from build123d import *

# Parameters (mm, degrees)
BOSS_EXTRUDE1_DEPTH = 6
SKETCH3_R           = 1.75
CUT_EXTRUDE1_DEPTH  = 84.570329663
SKETCH4_R           = 1.6
CUT_EXTRUDE2_DEPTH  = 81.721744282
FILLET1_R           = 3
FILLET2_R           = 1


with BuildPart() as part:
    # Sketch2 → Boss-Extrude1 (new body)
    with BuildSketch(Plane(origin=(0, 0, 0), x_dir=(1, 0, 0), z_dir=(0, 1, 0))):
        Polygon((6, -72), (12, -72), (12, -62), (19.625958238, -48.121978446), (30, -62), (30, -72), (36, -72), (36, -62), (0, -10), (0, 0), (-6, 0), (-6, -10), (12.471726571, -43.721673541), (6, -62), align=None)
    extrude(amount=BOSS_EXTRUDE1_DEPTH)

    # Sketch3 → Cut-Extrude1 (cut, through all)
    with BuildSketch(Plane(origin=(36, 0, 0), x_dir=(0, 0, -1), z_dir=(1, 0, 0))):
        with Locations((-67, 3)):
            Circle(SKETCH3_R)
    extrude(amount=-CUT_EXTRUDE1_DEPTH, mode=Mode.SUBTRACT)

    # Sketch4 → Cut-Extrude2 (cut, through all)
    with BuildSketch(Plane(origin=(0, 0, 0), x_dir=(0, 0, -1), z_dir=(1, 0, 0))):
        with Locations((-5, 3)):
            Circle(SKETCH4_R)
    extrude(amount=-CUT_EXTRUDE2_DEPTH, mode=Mode.SUBTRACT)

    # Fillet1
    fillet1_edges = [part.edges().sort_by_distance(p)[0] for p in [
        (-3, 0, 0),
        (-3, 6, 0),
        (33, 0, 72),
        (33, 6, 72),
        (9, 0, 72),
        (9, 6, 72),
    ]]
    fillet(fillet1_edges, radius=FILLET1_R - 0.0001)  # a hair under: the kernel refuses the full size

    # Fillet2
    fillet2_edges = [part.edges().sort_by_distance(p)[0] for p in [
        (0, 0, 6.49995),
        (18, 0, 36),
        (30, 0, 65.50005),
        (24.812979119, 0, 55.060989223),
        (15.812979119, 0, 55.060989223),
        (19.625958238, 3, 48.121978446),
        (12, 3, 62),
        (15.812979119, 6, 55.060989223),
        (24.812979119, 6, 55.060989223),
        (30, 6, 65.50005),
        (18, 6, 36),
        (0, 6, 6.49995),
        (-6, 0, 6.49995),
        (-6, 6, 6.49995),
        (-6, 5.121349633, 0.878650367),
        (-6, 0.878650367, 0.878650367),
        (36, 0, 65.50005),
        (12, 0, 65.50005),
        (0, 5.121349633, 0.878650367),
        (0, 0.878650367, 0.878650367),
        (12, 6, 65.50005),
        (36, 6, 65.50005),
        (36, 5.121349633, 71.121349633),
        (36, 0.878650367, 71.121349633),
        (30, 5.121349633, 71.121349633),
        (30, 0.878650367, 71.121349633),
        (12, 5.121349633, 71.121349633),
        (12, 0.878650367, 71.121349633),
    ]]
    fillet(fillet2_edges, radius=FILLET2_R)


solid = part.part
Input: part model. Units: mm. Frame: model coordinates. A direction names the side the tool comes from. Give positions to 0.01 mm unless a question says otherwise; leave off trailing zeros. Write each loop counter-clockwise with the first axis right and the second up, starting at its lowest first coordinate (ties: lowest second). Pieces come first, ordered by that corner, then holes. Notation, with made-up numbers: M -27,50 L -9,50 A30 cw -9,87 Z; hole C 31,10.5 d9. An arc over 180 degrees is marked long. Write item = value, one per line. Start each with the question number.
1) Cut plane B-B on z = 5. Return the cut outline in (x, y), then the cut area to 3 significant figures.
2) Draft query along X for faces 6 (the cylindrical face through (17.411, 5.715, 35.677)), 7 (the flat face through (25.21, 2.97, 55.59)), 8 (the cylindrical face through (33.03, 0.86, 71.1)). Return one class per face: +X half, -X half, draft (parallel to the pull), parting line (faces both ways), or undercut.
3) Cut plane A-A on z = 67. Return the cut outline in (x, y), then the cut area to 3 significant figures.
4) Reachability of faces 1 (the cylindrical face through (8.54, 0.9, 71.14)), 2 (the flat face through (9.281, 2.958, 52.733)), 3 (the flat face through (12, 1.6, 65.7)), 4 (the flat face through (6, 3, 65)), 5 (the flat face through (0, 3, 7)) from +Z, -Z, +X, -X, +Y, -Y: full face, straight path, thin tool, end or side. Return the list, or none.
5) First-contact query: pin 1 Ø3 at (x, y) = (29.5, 2) entering from +Z. Flat tip, straight axial feed; report the tip coordinate or a pass-through.
6) Material intervals for line 1 along Y through (x, z) = (-3.75, 5); line 2 along Y through (x, z) = (32, 67); line 3 along X through (y, z) = (0.5, 69), sorted ascending. Write a range as [from, to].
Solved:
q1.outline = M -6,1 A1 ccw -5,0 L -1,0 A1 ccw 0,1 L 0,1.4 L -6,1.4 Z; M -6,4.6 L 0,4.6 L 0,5 A1 ccw -1,6 L -5,6 A1 ccw -6,5 Z
q1.area = 15.9 mm2
q2.face_6 = +X half
q2.face_7 = undercut
q2.face_8 = draft
q3.outline = M 6,0 L 11,0 A1 ccw 12,1 L 12,1.25 L 6,1.25 Z; M 6,4.75 L 12,4.75 L 12,5 A1 ccw 11,6 L 6,6 Z; M 30,1 A1 ccw 31,0 L 35,0 A1 ccw 36,1 L 36,1.25 L 30,1.25 Z; M 30,4.75 L 36,4.75 L 36,5 A1 ccw 35,6 L 31,6 A1 ccw 30,5 Z
q3.area = 28.7 mm2
q4.face_1 = +Z, +X, -X, -Y
q4.face_2 = -X, +Y, -Y
q4.face_3 = +Z, +Y, -Y
q4.face_4 = +Z, -X, +Y, -Y
q4.face_5 = -Z, +X, +Y, -Y
q5.pin_1 = 71.97
q6.line_1 = [0, 1.4], [4.6, 6]
q6.line_2 = [0, 1.25], [4.75, 6]
q6.line_3 = [6, 11.87], [30.13, 35.87]
